from build123d import *

# Parameters (mm, degrees)
BOSS_EXTRUDE1_DEPTH                               = 12.7
CSK_FOR_6_FLAT_HEAD_MACHINE_SCREW_100_D           = 3.7973
CSK_FOR_6_FLAT_HEAD_MACHINE_SCREW_100_DEPTH       = 12.7
CSK_FOR_6_FLAT_HEAD_MACHINE_SCREW_100_CSINK_D     = 7.0866
CSK_FOR_6_FLAT_HEAD_MACHINE_SCREW_100_CSINK_ANGLE = 100
CSK_FOR_6_FLAT_HEAD_MACHINE_SCREW_100_TIP         = 1.140824014
F_6_0_204_DIAMETER_HOLE1_D                        = 5.1816
F_6_0_204_DIAMETER_HOLE1_DEPTH                    = 12.7
F_6_0_204_DIAMETER_HOLE1_TIP                      = 1.556709692


with BuildPart() as part:
    # Sketch1 → Boss-Extrude1 (new body)
    with BuildSketch(Plane.XY):
        Polygon((-1.5875, 19.05), (32.995567884, 39.016543552), (34.583067884, 36.266912895), (1.5875, 17.216912895), (1.5875, -19.05), (-1.5875, -19.05), align=None)
    extrude(amount=BOSS_EXTRUDE1_DEPTH)

    # CSK for #6 Flat Head Machine Screw (100)1
    with Locations(Plane(origin=(1.5875, 0, 0), x_dir=(0, 0, -1), z_dir=(1, 0, 0))):
        with Locations((-6.35, 7.247907124), (-6.35, -5.463667213)):
            CounterSinkHole(CSK_FOR_6_FLAT_HEAD_MACHINE_SCREW_100_D / 2, CSK_FOR_6_FLAT_HEAD_MACHINE_SCREW_100_CSINK_D / 2, depth=CSK_FOR_6_FLAT_HEAD_MACHINE_SCREW_100_DEPTH, counter_sink_angle=CSK_FOR_6_FLAT_HEAD_MACHINE_SCREW_100_CSINK_ANGLE)
            with Locations((0, 0, -(CSK_FOR_6_FLAT_HEAD_MACHINE_SCREW_100_DEPTH + CSK_FOR_6_FLAT_HEAD_MACHINE_SCREW_100_TIP / 2))):  # 118° drill point
                Cone(0, CSK_FOR_6_FLAT_HEAD_MACHINE_SCREW_100_D / 2, CSK_FOR_6_FLAT_HEAD_MACHINE_SCREW_100_TIP, mode=Mode.SUBTRACT)

    # #6 (0.204) Diameter Hole1
    with Locations(Plane(origin=(-7.058266971, 12.225277007, 0), x_dir=(-0.866025404, -0.5, 0), z_dir=(0.5, -0.866025404, 0))):
        with Locations((-43.476510232, -4.066670618), (-34.423038878, -9.068831988), (-25.680281164, -4.066670618), (-19.798832438, -9.068831988)):
            Hole(F_6_0_204_DIAMETER_HOLE1_D / 2, depth=F_6_0_204_DIAMETER_HOLE1_DEPTH)
            with Locations((0, 0, -(F_6_0_204_DIAMETER_HOLE1_DEPTH + F_6_0_204_DIAMETER_HOLE1_TIP / 2))):  # 118° drill point
                Cone(0, F_6_0_204_DIAMETER_HOLE1_D / 2, F_6_0_204_DIAMETER_HOLE1_TIP, mode=Mode.SUBTRACT)


solid = part.part
Part model, mm, in its own coordinate system. A direction names the side the tool comes from. Coordinates: 2 decimals unless noted, no trailing zeros. Order: outer loops, then holes, each group sorted by start corner. A loop starts at its lowest first (then second) coordinate and runs counter-clockwise, first axis right, second up.
(1) Probe L1, parallel to Y at x = -1.05, z = 6.35; L2, parallel to Y at x = -0.2, z = 6.35; L3, parallel to X at y = 15.5, z = 3.25. List the from-to ranges inside material, lowest first.
Check sheet entries:
L1: y = -19.05 to -7.36, -3.57 to 5.35, 9.15 to 19.36
L2: y = -19.05 to -7.36, -3.57 to 5.35, 9.15 to 19.85
L3: x = -1.59 to 1.59
(2) Slice it at B-B, the plane z = 7.5. State how many separate pieces and enclosed holes the cut face has, and give its area (3 significant figures).
Check sheet entries:
separate pieces: 5
enclosed holes: 0
area: 191 mm2
(3) Pin check, flat tips, straight feed: pin 1 Ø3 at (x, z) = (11, 8.5) entering from +Y; pin 2 Ø2 at (y, z) = (30.5, 1.5) entering from +X; pin 3 Ø1.5 at (x, z) = (15, 2) entering from -Y. Stop position of each tip, or through.
Check sheet entries:
pin 1: stops at y = 27.18
pin 2: stops at x = 26.33
pin 3: stops at y = 24.57
(4) Slice it at A-A, the plane y = 13. Write the cut outline in (x, z).
Check sheet entries:
outline: (-1.59, 0) - (1.59, 0) - (1.59, 12.7) - (-1.59, 12.7) - close
(5) Tool access for faces 1 (the face through (1.588, -1, 6)), 2 (the face through (7, 21, 12.7)): list every direction of +Z, -Z, +X, -X, +Y, -Y with a clear straight run to the whole face (end or side of a thin tool).
Check sheet entries:
face 1: +Z, -Z, +X, -Y
face 2: +Z, +X, -X, +Y, -Y
(6) Pull direction X, two halves, no side cores. Call faces 3 (the face through (15.462, 28.894, 6.261)), 4 (the face through (10.318, 24.117, 11.367)), 5 (the face through (-0.703, -7.148, 7.226)): pulls with the +X half, pulls with the -X half, needs draft (parallel to the pull), parting line crosses it, or undercut.
Check sheet entries:
face 3: pulls with the -X half
face 4: undercut
face 5: needs draft
